Verification items for the finished model (mm, model axes). A direction names the side the tool comes from. Round coordinates to 2 decimals unless told otherwise and drop trailing zeros. Write each loop counter-clockwise with the first axis right and the second up, starting at its lowest first coordinate (ties: lowest second). Pieces come first, ordered by that corner, then holes. Notation, with made-up numbers: M 26.25,80.5 L 55.25,80.5 A9 ccw 55.25,88.5 Z; hole C 64,57 d7. An arc over 180 degrees is marked long. One line per question, with ' | ' between items. Start each with the question number.
Q1. Gauge pin test, flat ends, axial feed: pin 1 (0.9 mm diameter, centred on x = 8, y = 4, fed in from +Z); pin 2 (8 mm diameter, centred on x = 15, z = -2, fed in from +Y); pin 3 (8 mm diameter, centred on x = 1, z = 7.5, fed in from +Y); pin 4 (1 mm diameter, centred on x = 2, y = 2, fed in from +Z). Record the tip position at first contact, or that the pin passes through.
Q2. Thickness scan on line 1 along X through (y, z) = (3.25, 0); line 2 along Y through (x, z) = (12, 8.5); line 3 along Y through (x, z) = (3.5, 1). Record the ranges inside material, lowest first. Write a range as from..to.
Q3. Release check for a two-part mould opening along X. For faces 6 (the face through (21, 3, 10)), 7 (the face through (26.07, 8.23, -0.07)), 8 (the face through (18.07, 8.23, -0.07)), 9 (the face through (4.56, 1.97, -2.92)) record: released by +X, released by -X, zero draft, split by the parting line, or undercut.
Q4. Cross-section at D-D (y = 1). Record the boundary of the cut face in (x, z), then the cut area to 3 significant figures.
Q5. Cross-section at C-C (x = 25.5). Record the boundary of the cut face in (y, z).
Q6. Cross-section at B-B (z = 0). Record the boundary of the cut face in (x, y), then the cut area to 3 significant figures.
Q7. Tool access check on faces 1 (the face through (4.464, 1.972, 2.945)), 2 (the face through (7.991, 5, 0)), 3 (the face through (21, 3, -10)), 4 (the face through (20.856, 8.232, -0.07)), 5 (the face through (0, 2, 0)). Record the directions out of +Z, -Z, +X, -X, +Y, -Y that give a thin tool (end or side, any length) a straight path to the whole face; none if there is none.
Q8. Cross-section at A-A (y = 5). Record the boundary of the cut face in (x, z), then the cut area to 3 significant figures.
from build123d import *

# Parameters (mm, degrees)
BOSS_EXTRUDE1_DEPTH     = 4
SKETCH2_R               = 3
CUT_EXTRUDE1_DEPTH      = 2
BOSS_EXTRUDE2_DEPTH     = 3
SKETCH24_W              = 20.502400247
SKETCH24_H              = 20
BOSS_EXTRUDE4_DEPTH     = 3
SKETCH26_W              = 3
SKETCH26_H              = 10
BOSS_EXTRUDE6_DEPTH     = 2.5
CUT_EXTRUDE2_DEPTH      = 10
CUT_EXTRUDE3_DEPTH      = 35.354616727
CUT_EXTRUDE3_DEPTH_BACK = 35.354616727


with BuildPart() as part:
    # Sketch1 → Boss-Extrude1 (new body)
    with BuildSketch(Plane(origin=(0, 0, 0), x_dir=(1, 0, 0), z_dir=(0, 1, 0))):
        with BuildLine():
            Line((31.464101615, 10), (10.961701368, 10))
            Line((10.961701368, 10), (9.668549449, 5.173891336))
            Line((9.668549449, 5.173891336), (8.818107828, 2))
            Line((8.818107828, 2), (7.990711605, 2))
            Line((7.990711605, 2), (1.03527618, 3.863703305))
            ThreePointArc((1.03527618, 3.863703305), (0.522104769, 3.965779445), (0, 4))
            ThreePointArc((0, 4), (-4, 0), (0, -4))
            ThreePointArc((0, -4), (0.522104769, -3.965779445), (1.03527618, -3.863703305))
            Line((1.03527618, -3.863703305), (7.990711605, -2))
            Line((7.990711605, -2), (8.818107828, -2))
            Line((8.818107828, -2), (9.668549449, -5.173891336))
            Line((9.668549449, -5.173891336), (10.961701368, -10))
            Line((10.961701368, -10), (31.464101615, -10))
            Line((31.464101615, -10), (31.464101615, 10))
        make_face()
    extrude(amount=BOSS_EXTRUDE1_DEPTH)

    # Sketch2 → Cut-Extrude1 (cut)
    with BuildSketch(Plane(origin=(0, 4, 0), x_dir=(1, 0, 0), z_dir=(0, 1, 0))):
        with Locations(Location((0, 0, 0), (0, 0, 270))):
            Circle(SKETCH2_R)
    extrude(amount=-CUT_EXTRUDE1_DEPTH, mode=Mode.SUBTRACT)

    # Sketch18 → Boss-Extrude2 (add)
    with BuildSketch(Plane(origin=(0, 4, 0), x_dir=(1, 0, 0), z_dir=(0, 1, 0))):
        Polygon((7.990711605, -2), (8.818107828, -2), (10.961701368, -10), (10.961701368, 10), (8.818107828, 2), (7.990711605, 2), align=None)
    extrude(amount=BOSS_EXTRUDE2_DEPTH)

    # Sketch24 → Boss-Extrude4 (add)
    with BuildSketch(Plane(origin=(0, 4, 0), x_dir=(1, 0, 0), z_dir=(0, 1, 0))):
        with Locations((21.212901491, 0)):
            Rectangle(SKETCH24_W, SKETCH24_H)
    extrude(amount=BOSS_EXTRUDE4_DEPTH)

    # Sketch26 → Boss-Extrude6 (add)
    with BuildSketch(Plane(origin=(0, 7, 0), x_dir=(1, 0, 0), z_dir=(0, 1, 0))):
        with Locations((27.464101615, 0)):
            Rectangle(SKETCH26_W, SKETCH26_H)
        with Locations((19.464101615, 0)):
            Rectangle(SKETCH26_W, SKETCH26_H)
    extrude(amount=BOSS_EXTRUDE6_DEPTH)

    # Sketch27 → Cut-Extrude2 (cut)
    with BuildSketch(Plane(origin=(0, 0, -5), x_dir=(-1, 0, 0), z_dir=(0, 0, -1))):
        Polygon((-28.964101615, 7), (-28.745379956, 9.5), (-28.964101615, 9.5), align=None)
        Polygon((-25.964101615, 7), (-26.182823274, 9.5), (-25.964101615, 9.5), align=None)
        Polygon((-20.964101615, 7), (-20.745379956, 9.5), (-20.964101615, 9.5), align=None)
        Polygon((-17.964101615, 7), (-18.182823274, 9.5), (-17.964101615, 9.5), align=None)
    extrude(amount=-CUT_EXTRUDE2_DEPTH, mode=Mode.SUBTRACT)

    # Sketch28 → Cut-Extrude3 (cut, two sides: drawn at the far end of the back side and taken through both)
    with BuildSketch(Plane(origin=(0, 0, 0), x_dir=(0, 0, -1), z_dir=(1, 0, 0)).offset(-CUT_EXTRUDE3_DEPTH_BACK)):
        Polygon((-5, 7), (-4.781278341, 9.5), (-5, 9.5), align=None)
        Polygon((5, 7), (4.781278341, 9.5), (5, 9.5), align=None)
    extrude(amount=CUT_EXTRUDE3_DEPTH + CUT_EXTRUDE3_DEPTH_BACK, mode=Mode.SUBTRACT)


solid = part.part
Determined:
1) pin 1: stops at z = 2.12 | pin 2: stops at y = 9.5 | pin 3: stops at y = 4 | pin 4: stops at z = 3.74
2) line 1: x = -4..-3, 3..31.46 | line 2: y = 0..7 | line 3: y = 0..4
3) face 6: zero draft | face 7: undercut | face 8: released by -X | face 9: undercut
4) outline: M 1.04,-3.86 L 7.99,-2 L 8.82,-2 L 10.96,-10 L 31.46,-10 L 31.46,10 L 10.96,10 L 8.82,2 L 7.99,2 L 1.04,3.86 A4 ccw long Z | area: 513 mm²
5) outline: M 0,-10 L 7,-10 L 7,10 L 0,10 Z
6) outline: M -4,0 L 31.46,0 L 31.46,7 L 28.96,7 L 28.75,9.5 L 26.18,9.5 L 25.96,7 L 20.96,7 L 20.75,9.5 L 18.18,9.5 L 17.96,7 L 7.99,7 L 7.99,4 L 3,4 L 3,2 L -3,2 L -3,4 L -4,4 Z | area: 214 mm²
7) face 1: +Z, +Y, -Y | face 2: +Z, -Z, -X, +Y | face 3: -Z, +X, -X, +Y, -Y | face 4: +Z, -Z, +Y | face 5: +Y
8) outline: M 7.99,-2 L 8.82,-2 L 10.96,-10 L 31.46,-10 L 31.46,10 L 10.96,10 L 8.82,2 L 7.99,2 Z | area: 439 mm²
